from build123d import *

# Parameters (mm, degrees)
SKICA1_R                 = 2
P_IDAT_VYSUNUT_M1_DEPTH  = 1
SKICA2_R                 = 1.15
ODEBRAT_VYSUNUT_M1_DEPTH = 2
SKICA3_R                 = 3
SKICA3_R_2               = 2
P_IDAT_VYSUNUT_M2_DEPTH  = 3


with BuildPart() as part:
    # Skica1 → Přidat vysunutím1 (new body)
    with BuildSketch(Plane(origin=(0, 0, 0), x_dir=(1, 0, 0), z_dir=(0, 1, 0))):
        with BuildLine():
            Line((-12.62, 1.495192295), (-2.5, 2.307395517))
            Line((-2.5, 2.307395517), (-2.5, 5.25))
            ThreePointArc((-2.5, 5.25), (0, 7.75), (2.5, 5.25))
            Line((2.5, 5.25), (2.5, 2.307395517))
            Line((2.5, 2.307395517), (12.62, 1.495192295))
            ThreePointArc((12.62, 1.495192295), (14, 0), (12.62, -1.495192295))
            Line((12.62, -1.495192295), (2.5, -2.307395517))
            Line((2.5, -2.307395517), (2.5, -5.25))
            ThreePointArc((2.5, -5.25), (0, -7.75), (-2.5, -5.25))
            Line((-2.5, -5.25), (-2.5, -2.307395517))
            Line((-2.5, -2.307395517), (-12.62, -1.495192295))
            ThreePointArc((-12.62, -1.495192295), (-14, 0), (-12.62, 1.495192295))
        make_face()
        Circle(SKICA1_R, mode=Mode.SUBTRACT)
    extrude(amount=P_IDAT_VYSUNUT_M1_DEPTH)

    # Skica2 → Odebrat vysunutím1 (cut)
    with BuildSketch(Plane(origin=(0, 1, 0), x_dir=(1, 0, 0), z_dir=(0, 1, 0))):
        with Locations((-8.5, 0)):
            Circle(SKICA2_R)
        with Locations((8.5, 0)):
            Circle(SKICA2_R)
    extrude(amount=-ODEBRAT_VYSUNUT_M1_DEPTH, mode=Mode.SUBTRACT)

    # Skica3 → Přidat vysunutím2 (add)
    with BuildSketch(Plane(origin=(0, 1, 0), x_dir=(1, 0, 0), z_dir=(0, 1, 0))):
        Circle(SKICA3_R)
        Circle(SKICA3_R_2, mode=Mode.SUBTRACT)
    extrude(amount=P_IDAT_VYSUNUT_M2_DEPTH)


solid = part.part
Geometry: final body of the model. Coordinates: model frame, mm. A direction names the side the tool comes from. Give positions to 0.01 mm unless a question says otherwise; leave off trailing zeros. Order: outer loops, then holes, each group sorted by start corner. A loop starts at its lowest first (then second) coordinate and runs counter-clockwise, first axis right, second up. Notation, with made-up numbers: (26, -26.75) -> (49, -26.75) arc R24 cw to (49, -7.75) -> close; hole circle Ø4 at (-15.75, 56). An arc over 180 degrees is marked (long way). Answer as a JSON object with one key per item and string values.
Q1. Draft query along X for faces 4 (the cylindrical face through (0, 2, 2)), 5 (the cylindrical face through (-3, 2, 0)), 6 (the flat face through (7.6, 0.5, 1.9)). Return one class per face: released by +X, released by -X, zero draft, split by the parting line, or undercut.
Entries:
{"face 4": "undercut", "face 5": "split by the parting line", "face 6": "released by +X"}
Q2. Section A-A (z = 0). Output: boundary loops of the cut face in (x, y).
Entries:
{"outline": "(-14, 0) -> (-9.65, 0) -> (-9.65, 1) -> (-14, 1) -> close; (-7.35, 0) -> (-2, 0) -> (-2, 4) -> (-3, 4) -> (-3, 1) -> (-7.35, 1) -> close; (2, 0) -> (7.35, 0) -> (7.35, 1) -> (3, 1) -> (3, 4) -> (2, 4) -> close; (9.65, 0) -> (14, 0) -> (14, 1) -> (9.65, 1) -> close"}
Q3. Material intervals for probe 1 along Z at (x, y) = (0, 1.2); probe 2 along Y at (x, z) = (11.5, 1.5), sorted ascending.
Entries:
{"probe 1": "z = -3 to -2, 2 to 3", "probe 2": "y = 0 to 1"}
Q4. Section C-C (y = 0.3). Output: boundary loops of the cut face in (x, z), plus the area to 3 significant figures.
Entries:
{"outline": "(-12.62, -1.5) -> (-2.5, -2.31) -> (-2.5, -5.25) arc R2.5 ccw to (2.5, -5.25) -> (2.5, -2.31) -> (12.62, -1.5) arc R1.5 ccw to (12.62, 1.5) -> (2.5, 2.31) -> (2.5, 5.25) arc R2.5 ccw to (-2.5, 5.25) -> (-2.5, 2.31) -> (-12.62, 1.5) arc R1.5 ccw to start; hole circle Ø2.3 at (-8.5, 0); hole circle Ø4 at (0, 0); hole circle Ø2.3 at (8.5, 0)", "area": "135 mm^2"}
Q5. Section D-D (y = 3.7). Output: boundary loops of the cut face in (x, z).
Entries:
{"outline": "circle Ø6 at (0, 0); hole circle Ø4 at (0, 0)"}
Q6. Access query for faces 1 (the flat face through (2.5, 0.5, -3.8)), 2 (the flat face through (-3, 1, 1)), 3 (the flat face through (-2.5, 0.5, 3.8)). Directions: +Z, -Z, +X, -X, +Y, -Y. A direction counts if a zero-diameter tool reaches every point of the face in a straight line with its end or side. Return the directions, or none.
Entries:
{"face 1": "-Z, +X, +Y, -Y", "face 2": "+Y", "face 3": "+Z, -X, +Y, -Y"}
Q7. First-contact query: pin 1 (1.1 mm diameter, centred on y = 0.5, z = -4, fed in from +X); pin 2 (2 mm diameter, centred on x = -8.5, z = 0, fed in from -Y); pin 3 (3 mm diameter, centred on x = 8.5, z = 0, fed in from +Y); pin 4 (1.5 mm diameter, centred on y = 2, z = 2, fed in from -X). Flat tips, straight axial feed; report the tip coordinate or a pass-through.
Entries:
{"pin 1": "stops at x = 2.5", "pin 2": "passes through", "pin 3": "stops at y = 1", "pin 4": "stops at x = -2.73"}
Q8. Section B-B (x = 0). Output: boundary loops of the cut face in (y, z).
Entries:
{"outline": "(0, -7.75) -> (1, -7.75) -> (1, -3) -> (4, -3) -> (4, -2) -> (0, -2) -> close; (0, 2) -> (4, 2) -> (4, 3) -> (1, 3) -> (1, 7.75) -> (0, 7.75) -> close"}
